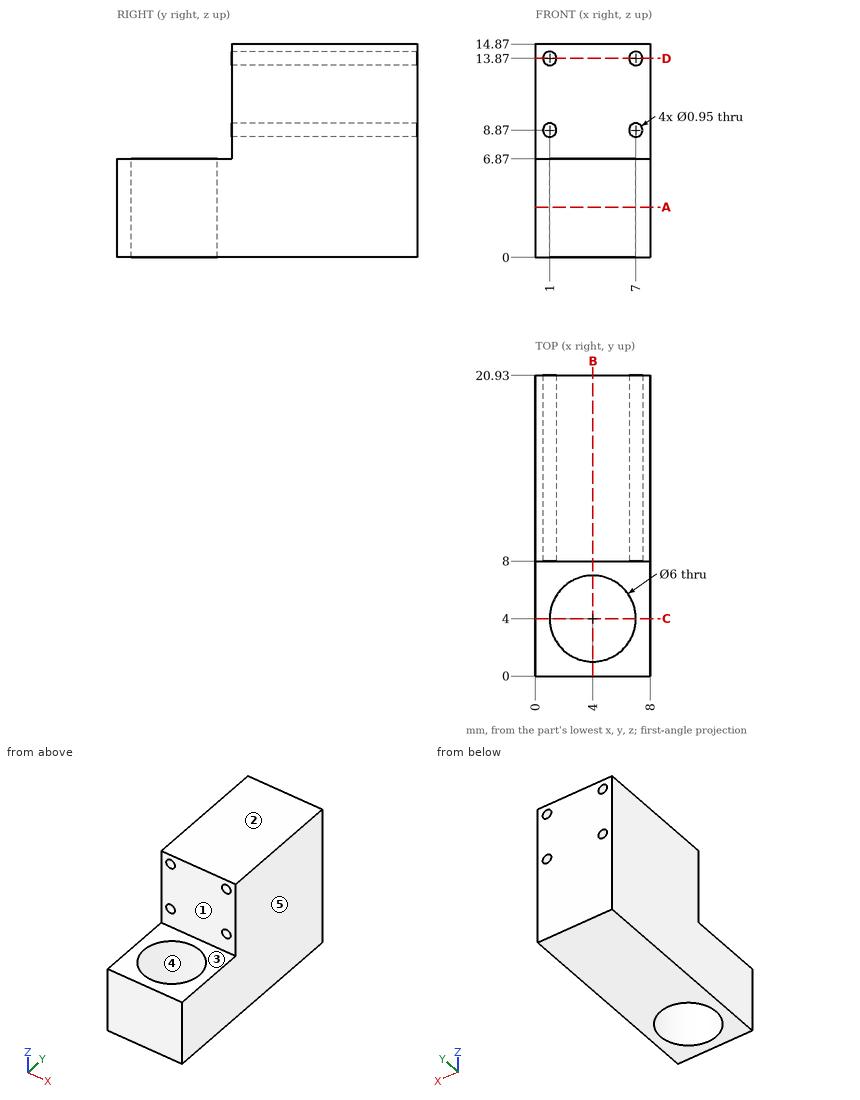
Input: dimensioned drawing with shaded views. Units: mm. Origin: part minimum x, y, z. A direction names the side the tool comes from. Round coordinates to 2 decimals unless told otherwise and drop trailing zeros. Loops run counter-clockwise (first coordinate to the right, second up) from the corner with the lowest first, then second, coordinate; pieces in that order, holes last. Notation, with made-up numbers: (78.25, 56) -> (106.25, 56) arc R12 cw to (106.25, 66) -> close; hole circle Ø2 at (74, 63). An arc over 180 degrees is marked (long way). Use one line per item in the form item = value. Start each with the question number.
1) Access query for the marked faces 1 and 2. Directions: +Z, -Z, +X, -X, +Y, -Y. A direction counts if a zero-diameter tool reaches every point of the face in a straight line with its end or side. Return the directions, or none.
2) First-contact query: P1, Ø5, axis at y = 13, z = 11, coming from the -X side. Flat tip, straight axial feed; report the tip coordinate or a pass-through.
3) Line query: L1, parallel to Z at x = 7, y = 16.25 (3 decimals); L2, parallel to X at y = 14.75, z = 14.25 (3 decimals); L3, parallel to Y at x = 4, z = 2.75. Output: solid intervals per line, ascending.
4) Section D-D on z = 13.87. Output: boundary loops of the cut face in (x, y) (3 decimals), then the cut area to 3 significant figures.
5) Section B-B on x = 4. Output: boundary loops of the cut face in (y, z), then the cut area to 3 significant figures.
6) Section A-A on z = 3.5. Output: boundary loops of the cut face in (x, y).
7) Draft query along X for the marked faces 3, 4 and 5. Return one class per face: released by +X, released by -X, zero draft, split by the parting line, or undercut.
8) Section C-C on y = 4. Output: boundary loops of the cut face in (x, z).
Response:
q1.face_1 = +Z, +X, -X, -Y
q1.face_2 = +Z, +X, -X, +Y, -Y
q2.P1 = 0
q3.L1 = 0 to 8.395, 9.345 to 13.395, 14.345 to 14.87
q3.L2 = 0 to 0.715, 1.285 to 6.715, 7.285 to 8
q3.L3 = 0 to 1, 7 to 20.93
q4.outline = (0, 8) -> (0.525, 8) -> (0.525, 20.93) -> (0, 20.93) -> close; (1.475, 8) -> (6.525, 8) -> (6.525, 20.93) -> (1.475, 20.93) -> close; (7.475, 8) -> (8, 8) -> (8, 20.93) -> (7.475, 20.93) -> close
q4.area = 78.9 mm^2
q5.outline = (0, 0) -> (1, 0) -> (1, 6.87) -> (0, 6.87) -> close; (7, 0) -> (20.93, 0) -> (20.93, 14.87) -> (8, 14.87) -> (8, 6.87) -> (7, 6.87) -> close
q5.area = 206 mm^2
q6.outline = (0, 0) -> (8, 0) -> (8, 20.93) -> (0, 20.93) -> close; hole circle Ø6 at (4, 4)
q7.face_3 = zero draft
q7.face_4 = undercut
q7.face_5 = released by +X
q8.outline = (0, 0) -> (1, 0) -> (1, 6.87) -> (0, 6.87) -> close; (7, 0) -> (8, 0) -> (8, 6.87) -> (7, 6.87) -> close
